Here's how the part is built. I have some questions about the finished solid (model axes, mm). Face numbers are marked on the shaded views. A direction names the side the tool comes from. Give positions to 0.01 mm unless a question says otherwise; leave off trailing zeros. Order: outer loops, then holes, each group sorted by start corner. A loop starts at its lowest first (then second) coordinate and runs counter-clockwise, first axis right, second up. Notation, with made-up numbers: M 77.5,64.5 L 95.5,64.5 A20 cw 95.5,86.5 Z; hole C 14,59.5 d11. An arc over 180 degrees is marked long. Use one line per item in the form item = value.
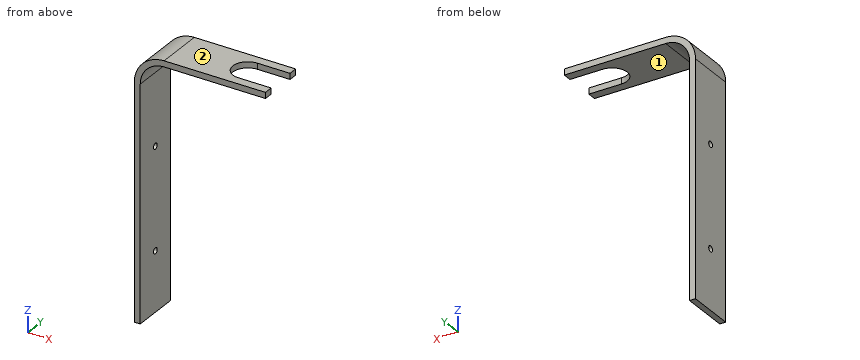
from build123d import *

# Parameters (mm, degrees)
F1_DEPTH = 12.7
F3_DEPTH = 25.4
F4_R     = 1.5875
F5_DEPTH = 25.4


with BuildPart() as f1:
    # F0 (on Front) → F1 (new body, symmetric)
    with BuildSketch(Plane.XZ):
        with BuildLine():
            Line((69.85, 0), (15.875, 0))
            ThreePointArc((15.875, 0), (4.64968, -4.64968), (0, -15.875))
            Line((0, -15.875), (0, -139.7))
            Line((0, -139.7), (3.175, -139.7))
            Line((3.175, -139.7), (3.175, -15.875))
            ThreePointArc((3.175, -15.875), (6.894744, -6.894744), (15.875, -3.175))
            Line((15.875, -3.175), (69.85, -3.175))
            Line((69.85, -3.175), (69.85, 0))
        make_face()
    extrude(amount=F1_DEPTH, both=True)

    # F2 (on face) → F3 (cut)
    with BuildSketch(Plane.XY):
        with BuildLine():
            ThreePointArc((52.3875, -7.9375), (58.00016, -5.61266), (60.325, 0))
            ThreePointArc((60.325, 0), (58.00016, 5.61266), (52.3875, 7.9375))
            ThreePointArc((52.3875, 7.9375), (44.45, 0), (52.3875, -7.9375))
        make_face()
        with BuildLine():
            ThreePointArc((52.3875, 7.9375), (58.00016, 5.61266), (60.325, 0))
            ThreePointArc((60.325, 0), (58.00016, -5.61266), (52.3875, -7.9375))
            Line((52.3875, -7.9375), (69.85, -7.9375))
            Line((69.85, -7.9375), (69.85, 7.9375))
            Line((69.85, 7.9375), (52.3875, 7.9375))
        make_face()
    extrude(amount=-F3_DEPTH, mode=Mode.SUBTRACT)

    # F4 (on face) → F5 (cut)
    with BuildSketch(Plane(origin=(0, 0, 0), x_dir=(0, -1, 0), z_dir=(-1, 0, 0))):
        with Locations((0, -53.975)):
            Circle(F4_R)
        with Locations((0, -107.95)):
            Circle(F4_R)
    extrude(amount=-F5_DEPTH, mode=Mode.SUBTRACT)


solid = f1.part
Q1. I want a section at B-B on y = 0. State how many separate pieces and enclosed holes the cut face has, then the cut area to 3 significant figures.
Found:
separate_pieces = 3
enclosed_holes = 0
area = 535 mm²
Q2. On a 3-axis mill with a long thin cutter (end or side, diameter ignored), from which of +Z, -Z, +X, -X, +Y, -Y can I reach the whole of each face in a straight line? I mean the marked faces 1 and 2. Say none if no direction works.
Found:
face_1 = -Z, +X, +Y, -Y
face_2 = +Z, +X, -X, +Y, -Y
Q3. I want a section at C-C on z = -107.95. Write out the boundary of the cut face in (x, y) (1 decimal).
Found:
outline = M 0,-12.7 L 3.2,-12.7 L 3.2,-1.6 L 0,-1.6 Z; M 0,1.6 L 3.2,1.6 L 3.2,12.7 L 0,12.7 Z
Q4. I'm going to push flat-ended pins straight in: pin 1 Ø2 at (y, z) = (-5.5, -14.5) entering from +X; pin 2 Ø5 at (y, z) = (-7, -45.5) entering from +X (3 decimals); pin 3 Ø3 at (y, z) = (0, -53.975) entering from +X; pin 4 Ø10 at (x, y) = (37, 1) entering from -Z (3 decimals). Where does each tip first touch, or does it pass through?
Found:
pin_1 = 3.4
pin_2 = 3.175
pin_3 = through
pin_4 = -3.175
Q5. I want a section at D-D on y = -10.5. Write out the boundary of the cut face in (x, z) (3 decimals), then the cut area to 3 significant figures.
Found:
outline = M 0,-139.7 L 3.175,-139.7 L 3.175,-15.875 A12.7 cw 15.875,-3.175 L 69.85,-3.175 L 69.85,0 L 15.875,0 A15.875 ccw 0,-15.875 Z
area = 636 mm²
Q6. I want a section at A-A on x = 59.5. Write out the boundary of the cut face in (y, z) (1 decimal), then the cut area to 3 significant figures.
Found:
outline = M -12.7,-3.2 L -7.9,-3.2 L -7.9,0 L -12.7,0 Z; M 7.9,-3.2 L 12.7,-3.2 L 12.7,0 L 7.9,0 Z
area = 30.2 mm²
Q7. I need wall thicknesses on L1, parallel to Y at x = 1.6, z = -107.95; L2, parallel to Z at x = 1.8, y = 0; L3, parallel to Z at x = 2.05, y = 0. Which ranges of each line are inside material? Lowest first, please.
Found:
L1 = -12.7 to -1.59, 1.59 to 12.7
L2 = -139.7 to -109.54, -106.36 to -55.56, -52.39 to -8.53
L3 = -139.7 to -109.54, -106.36 to -55.56, -52.39 to -8.07
